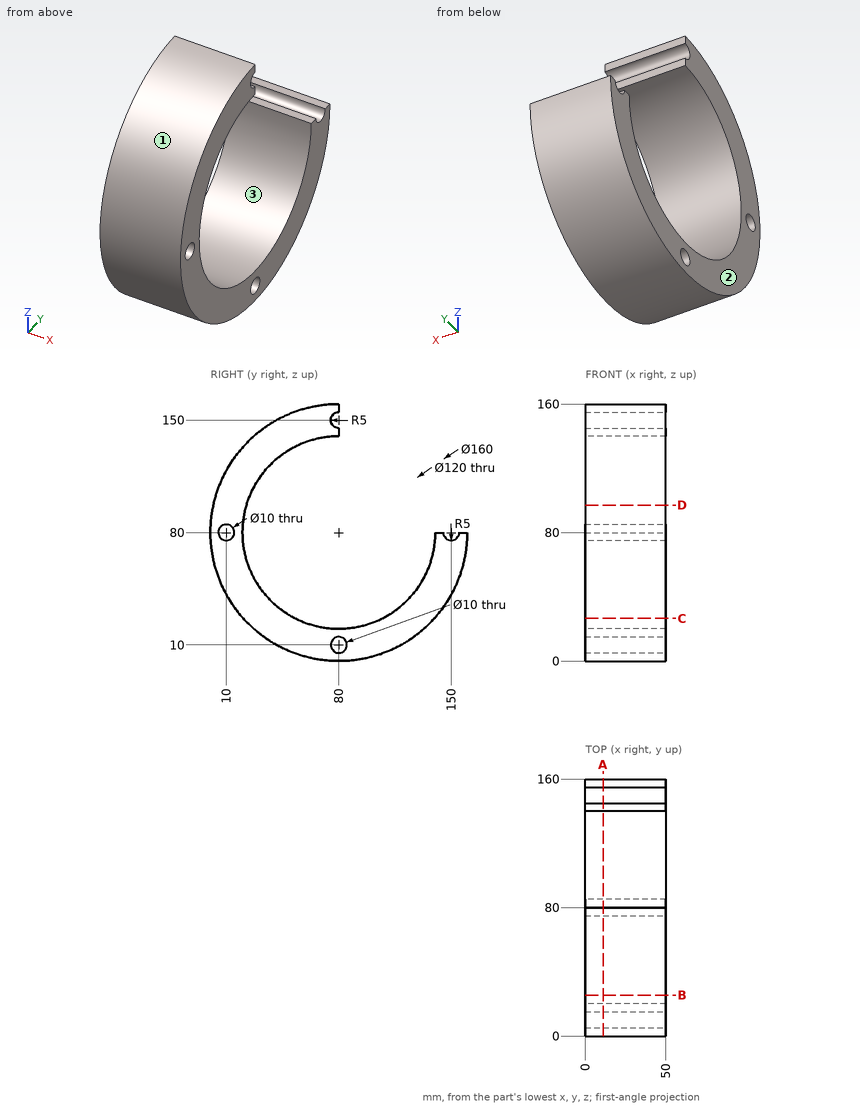
Here's the drawing with two shaded views (mm, measured from the low corner). I have some questions. Coordinates: 2 decimals unless noted, no trailing zeros. Loops run counter-clockwise (first coordinate to the right, second up) from the corner with the lowest first, then second, coordinate; pieces in that order, holes last. Notation, with made-up numbers: (-38, 51) -> (0, 51) arc R22 cw to (0, 86) -> close; hole circle Ø5 at (0.5, -14.75). An arc over 180 degrees is marked (long way). Answer as a JSON object with one key per item and string values.
1) Imagine slicing it at A-A (x = 11). Please give me the cut outline in (y, z).
Results:
{"outline": "(80, 140) -> (80, 145) arc R5 cw to (80, 155) -> (80, 160) arc R80 ccw (long way) to (160, 80) -> (155, 80) arc R5 cw to (145, 80) -> (140, 80) arc R60 cw (long way) to start; hole circle Ø10 at (10, 80); hole circle Ø10 at (80, 10)"}
2) Imagine slicing it at C-C (z = 26.5). Please give me the cut outline in (x, y), then the cut area to 3 significant figures.
Results:
{"outline": "(0, 20.52) -> (50, 20.52) -> (50, 52.84) -> (0, 52.84) -> close; (0, 107.16) -> (50, 107.16) -> (50, 139.48) -> (0, 139.48) -> close", "area": "3,230 mm^2"}
3) Imagine slicing it at D-D (z = 97). Please give me the cut outline in (x, y), then the cut area to 3 significant figures.
Results:
{"outline": "(0, 1.83) -> (50, 1.83) -> (50, 22.46) -> (0, 22.46) -> close", "area": "1,030 mm^2"}
4) For P1, Ø1.5, axis at x = 18.5, z = 158, coming from the +Y side; P2, Ø1.5, axis at x = 32, y = 157.5, coming from the +Z side; P3, Ø10, axis at x = 16, z = 92.5, coming from the -Y side, each with a flat end and sliding along its axis, tell me the tip position at first contact or that it passes through.
Results:
{"P1": "stops at y = 80", "P2": "stops at z = 80", "P3": "stops at y = 0.35"}
5) Imagine slicing it at B-B (y = 25.5). Please give me the cut outline in (x, z).
Results:
{"outline": "(0, 21.44) -> (50, 21.44) -> (50, 54.91) -> (0, 54.91) -> close; (0, 105.09) -> (50, 105.09) -> (50, 138.56) -> (0, 138.56) -> close"}
6) Thinking about a two-plate mould opening in Z: for the marked faces 1, 2 and 3, which applies, pulls with the +Z half, pulls with the -Z half, needs draft (parallel to the pull), parting line crosses it, or undercut?
Results:
{"face 1": "parting line crosses it", "face 2": "needs draft", "face 3": "undercut"}
7) If I drill on line 1 (Z direction, x = 30, y = 79); line 2 (Y direction, x = 22.5, z = 29.5); line 3 (Y direction, x = 4, z = 26), over which ranges is the centre line in solid material (lowest first)?
Results:
{"line 1": "z = 0.01 to 5.1, 14.9 to 20.01, 139.99 to 145.1, 154.9 to 159.99", "line 2": "y = 17.95 to 47.6, 112.4 to 142.05", "line 3": "y = 20.97 to 53.85, 106.15 to 139.03"}
